Geometry check sheet. Reference: the model listing, model coordinates, mm. A direction names the side the tool comes from. Round coordinates to 2 decimals unless told otherwise and drop trailing zeros. Order: outer loops, then holes, each group sorted by start corner. A loop starts at its lowest first (then second) coordinate and runs counter-clockwise, first axis right, second up.
(1) Thickness scan on L1, parallel to Y at x = 9.5, z = -14; L2, parallel to X at y = 9.5, z = -1; L3, parallel to Z at x = -2, y = 2.25. Record the ranges inside material, lowest first.
(2) Draft check along X on faces 4 (the face through (-5.48, 6.44, -3.11)), 5 (the face through (-5.43, 6.44, 3.2)), 6 (the face through (-1.74, 8.84, 13.22)), 7 (the face through (6, 12.7, 3)). Enter one of: pulls with the +X half, pulls with the -X half, needs draft (parallel to the pull), parting line crosses it, or undercut.
(3) Gauge pin test, flat ends, axial feed: P1, Ø1.5, axis at x = -4, z = -1.5, coming from the +Y side; P2, Ø3, axis at x = -1, z = -13.5, coming from the -Y side; P3, Ø2, axis at x = 0, y = 7.5, coming from the +Z side (3 decimals); P4, Ø2, axis at x = 5.5, y = 3.5, coming from the +Z side. Record the tip position at first contact, or that the pin passes through.
(4) Cross-section at A-A on y = 11.75. Enter the section's corners in (x, z) (3 decimals).
(5) Cross-section at D-D on z = 9. Enter the section's corners in (x, y).
(6) Cross-section at B-B on z = -2.5. Enter the section's corners in (x, y), and give its area (3 significant figures).
(7) Cross-section at C-C on x = 0. Enter the section's corners in (y, z) (3 decimals), and give its area (3 significant figures).
(8) Set-up check for faces 1 (the face through (5.48, 6.44, 3.11)), 2 (the face through (-7.4, 0, 0.2)), 3 (the face through (10.24, 5.08, -8.81)): record each of +Z, -Z, +X, -X, +Y, -Y from which the full face is reachable in a straight line by a thin tool's end or side.
Autodesk Inventor part; units mm, degrees
ref_plane "YZ Plane" through (0, 0, 0) normal (1, 0, 0) x (0, 1, 0)
ref_plane "XZ Plane" through (0, 0, 0) normal (0, 1, 0) x (-1, 0, 0)
ref_plane "XY Plane" through (0, 0, 0) normal (0, 0, 1) x (1, 0, 0)
sketch "Sketch1" plane through (0, 0, 0) normal (0, 1, 0) x (-1, 0, 0)
  circle A0 centre (0, 0) radius 17.145
  dimension "d0" = 34.29
extrude "Extrusion1" add sketch "Sketch1" along normal blind 5.08
sketch "Sketch2" plane through (0, 5.08, 0) normal (0, 1, 0) x (1, 0, 0)
  circle A0 centre (0, 0) radius 13.335
  dimension "d3" = 26.67
extrude "Extrusion2" add sketch "Sketch2" along normal blind 7.62
sketch "Sketch3" plane through (0, 12.7, 0) normal (0, 1, 0) x (1, 0, 0)
  line L0 (-3.6383, -6.3018) -> (-7.2767, 0)
  line L1 (-7.2767, 0) -> (-3.6383, 6.3018)
  line L2 (-3.6383, 6.3018) -> (3.6383, 6.3018)
  line L3 (3.6383, 6.3018) -> (7.2767, 0)
  line L4 (7.2767, 0) -> (3.6383, -6.3018)
  line L5 (3.6383, -6.3018) -> (-3.6383, -6.3018)
  point P0 (0, 0)
  point P1 (0, 0)
extrude "Extrusion3" cut sketch "Sketch3" against normal blind 12.7
properties part number "Hex Shaft Holder"
Found:
1. L1: y = 0 to 5.08
1. L2: x = -13.3 to -6.7, 6.7 to 13.3
1. L3: z = -17.03 to -6.3, 6.3 to 17.03
2. face 4: undercut
2. face 5: undercut
2. face 6: parting line crosses it
2. face 7: needs draft
3. P1: passes through
3. P2: stops at y = 0
3. P3: stops at z = 13.335
3. P4: stops at z = 16.54
4. outline: circle Ø26.67 at (0, 0); hole (-7.277, 0) - (-3.638, -6.302) - (3.638, -6.302) - (7.277, 0) - (3.638, 6.302) - (-3.638, 6.302) - close
5. outline: (-14.59, 0) - (14.59, 0) - (14.59, 5.08) - (9.84, 5.08) - (9.84, 12.7) - (-9.84, 12.7) - (-9.84, 5.08) - (-14.59, 5.08) - close
6. outline: (-16.96, 0) - (-5.83, 0) - (-5.83, 12.7) - (-13.1, 12.7) - (-13.1, 5.08) - (-16.96, 5.08) - close; (5.83, 0) - (16.96, 0) - (16.96, 5.08) - (13.1, 5.08) - (13.1, 12.7) - (5.83, 12.7) - close
6. area: 224 mm2
7. outline: (0, -17.145) - (5.08, -17.145) - (5.08, -13.335) - (12.7, -13.335) - (12.7, -6.302) - (0, -6.302) - close; (0, 6.302) - (12.7, 6.302) - (12.7, 13.335) - (5.08, 13.335) - (5.08, 17.145) - (0, 17.145) - close
7. area: 217 mm2
8. face 1: +Y, -Y
8. face 2: +Z, -Z, +X, -X, -Y
8. face 3: +Y
